```python
from build123d import *

# Parameters (mm, degrees)
F0_W      = 197.231
F0_H      = 140.208
F1_DEPTH  = 73.025
F2_R      = 10.16
F3_T      = -2.54
F4_W      = 11.0265567622
F4_H      = 70.485
F4_W_2    = 137.668
F5_DEPTH  = 25.4
F6_R      = 5.08
F7_W      = 127.508
F7_H      = 60.1236441541
F8_DEPTH  = 25.4
F10_DEPTH = 254


with BuildPart() as f1:
    # F0 (on Top) → F1 (new body)
    with BuildSketch(Plane.XY):
        Rectangle(F0_W, F0_H)
    extrude(amount=F1_DEPTH)

    # F2
    f2_edges = [f1.edges().sort_by_distance(p)[0] for p in [
        (98.6155, 0, 73.025),
    ]]
    fillet(f2_edges, radius=F2_R)

    # F3
    f3_openings = [f1.faces().sort_by_distance(p)[0] for p in [
        (0, 0, 0),
    ]]
    offset(amount=F3_T, openings=f3_openings)

    # F4 (on face) → F5 (cut)
    with BuildSketch(Plane(origin=(-98.6155, 0, 0), x_dir=(0, -1, 0), z_dir=(-1, 0, 0))):
        with Locations((-75.6172783811, 35.2425)):
            Rectangle(F4_W, F4_H)
        with Locations((-1.27, 35.2425)):
            Rectangle(F4_W_2, F4_H)
    extrude(amount=-F5_DEPTH, mode=Mode.SUBTRACT)

    # F6
    f6_edges = [f1.edges().sort_by_distance(p)[0] for p in [
        (96.0755, -67.564, 31.4325),
        (96.0755, 67.564, 31.4325),
    ]]
    fillet(f6_edges, radius=F6_R)

    # F7 (on face) → F8 (cut)
    with BuildSketch(Plane.YZ.offset(98.6155)):
        with Locations((0, 30.061822077)):
            Rectangle(F7_W, F7_H)
    extrude(amount=-F8_DEPTH, mode=Mode.SUBTRACT)

    # F9 (on face) → F10 (cut)
    with BuildSketch(Plane.XZ.offset(70.104)):
        with BuildLine():
            Line((-98.6155, 70.485), (-98.6155, 0))
            Line((-98.6155, 0), (-16.0655, 0))
            Line((-16.0655, 0), (-13.1894074903, 63.8492537147))
            ThreePointArc((-13.1894074903, 63.8492537147), (-14.9429320556, 68.5229386441), (-19.5329750245, 70.485))
            Line((-19.5329750245, 70.485), (-98.6155, 70.485))
        make_face()
    extrude(amount=-F10_DEPTH, mode=Mode.SUBTRACT)


solid = f1.part
```
Check sheet for the modelled part. Datum: model origin and axes. Units: mm. A direction names the side the tool comes from. Coordinates: 2 decimals unless noted, no trailing zeros. Loops run counter-clockwise (first coordinate to the right, second up) from the corner with the lowest first, then second, coordinate; pieces in that order, holes last.
1) Access from +Z, -Z, +X, -X, +Y, -Y to the whole of each face (thin tool, end or side, straight path). Record for faces 5 (the face through (93.955, -66.613, 31.873)), 6 (the face through (-6, 1, 73.025)).
2) Release check for a two-part mould opening along Z. For faces 1 (the face through (33.705, -66.036, 69.036)), 2 (the face through (-15.7, 67.9, 69.2)), 3 (the face through (37, 67.564, 32)), 4 (the face through (-15.7, -68, 69.2)) record: released by +Z, released by -Z, zero draft, split by the parting line, or undercut.
3) Sectioned sample at B-B (z = 49). Record the boundary of the cut face in (x, y), and give its area (3 significant figures).
4) Gauge pin test, flat ends, axial feed: pin 1 (1.5 mm diameter, centred on x = -39, y = -26.5, fed in from -Z) (3 decimals); pin 2 (1.4 mm diameter, centred on x = 97.5, y = -6.5, fed in from -Z); pin 3 (0.8 mm diameter, centred on y = -27.5, z = 62, fed in from -X). Record the tip position at first contact, or that the pin passes through.
5) Sectioned sample at C-C (x = 38). Record the boundary of the cut face in (y, z) (3 decimals).
6) Sectioned sample at D-D (z = 12.5). Record the boundary of the cut face in (x, y), and give its area (3 significant figures).
7) Material ranges on probe 1 along Y at (x, z) = (3, 36.5); probe 2 along Z at (x, y) = (26.5, 4) (3 decimals); probe 3 along Z at (x, y) = (82.5, 63.5) (3 decimals), recorded low to high.
8) Sectioned sample at A-A (y = -21). Record the boundary of the cut face in (x, z) (1 decimal).
Check sheet entries:
1. face 5: -Z, -X
1. face 6: +Z, +X, -X, +Y, -Y
2. face 1: released by -Z
2. face 2: undercut
2. face 3: zero draft
2. face 4: undercut
3. outline: (-13.86, -70.1) - (98.62, -70.1) - (98.62, -63.75) - (95.91, -63.75) arc R5.08 cw to (91, -67.56) - (-13.86, -67.56) - close; (-13.86, 67.56) - (91, 67.56) arc R5.08 cw to (95.91, 63.75) - (98.62, 63.75) - (98.62, 70.1) - (-13.86, 70.1) - close
3. area: 602 mm2
4. pin 1: stops at z = 70.485
4. pin 2: stops at z = 60.12
4. pin 3: stops at x = 96.08
5. outline: (-70.104, 0) - (-67.564, 0) - (-67.564, 65.405) arc R5.08 cw to (-62.484, 70.485) - (62.484, 70.485) arc R5.08 cw to (67.564, 65.405) - (67.564, 0) - (70.104, 0) - (70.104, 73.025) - (-70.104, 73.025) - close
6. outline: (-15.5, -70.1) - (98.62, -70.1) - (98.62, -63.75) - (95.91, -63.75) arc R5.08 cw to (91, -67.56) - (-15.5, -67.56) - close; (-15.5, 67.56) - (91, 67.56) arc R5.08 cw to (95.91, 63.75) - (98.62, 63.75) - (98.62, 70.1) - (-15.5, 70.1) - close
6. area: 610 mm2
7. probe 1: y = -70.1 to -67.56, 67.56 to 70.1
7. probe 2: z = 70.485 to 73.025
7. probe 3: z = 70.382 to 73.025
8. outline: (-98.6, 70.5) - (88.5, 70.5) arc R7.6 cw to (96.1, 62.9) - (96.1, 60.1) - (98.6, 60.1) - (98.6, 62.9) arc R10.2 ccw to (88.5, 73) - (-98.6, 73) - close
